Part model, mm, in its own coordinate system. Round coordinates to 2 decimals unless told otherwise and drop trailing zeros. Use CSV: the item, a comma, the result in double quotes. Start each with the question number.
```python
from build123d import *


with BuildPart() as part:
    # Sweep1: sweep along a path in Sketch4
    with BuildLine(Plane.XY) as sweep1_path:
        ThreePointArc((0, 0), (-12.933123295, 3.638699735), (-23.377708341, 12.089525561))
        ThreePointArc((-23.377708341, 12.089525561), (-38.1, 19.05), (-52.822291659, 12.089525561))
        ThreePointArc((-52.822291659, 12.089525561), (-63.266876705, 3.638699735), (-76.2, 0))
    # Sketch2 → Sweep1 (sweep)
    with BuildSketch(Plane(origin=(0, 0, 0), x_dir=(0, 0, -1), z_dir=(1, 0, 0))):
        with BuildLine():
            ThreePointArc((14.885260382, -2.399980647), (0, 2.544792821), (-14.885260382, -2.399980647))
            ThreePointArc((-14.885260382, -2.399980647), (-16.662734914, -2.14232916), (-16.405083427, -0.364854628))
            ThreePointArc((-16.405083427, -0.364854628), (0, 5.084792821), (16.405083427, -0.364854628))
            ThreePointArc((16.405083427, -0.364854628), (16.662734914, -2.14232916), (14.885260382, -2.399980647))
        make_face()
    sweep(path=sweep1_path.line)


solid = part.part
```
1. Drill centre lines: line 1 along X through (y, z) = (7.25, 7); line 2 along Z through (x, y) = (-11.5, 0.5); line 3 along X through (y, z) = (11.75, 13.5). Where is each one in solid material? Low to high. Write a range as [from, to].
2. Band-saw the part on A-A (y = 0.75). Give the number of separate pieces and of enclosed holes in the cut face, then the cut area to 3 significant figures.
3. Flat gauge pins, fed straight in: pin 1 (4 mm diameter, centred on x = -31.5, z = -7.5, fed in from -Y); pin 2 (3 mm diameter, centred on y = 15.5, z = -3, fed in from +X); pin 3 (12 mm diameter, centred on x = -24.5, z = -5, fed in from +Y). Where does each tip first touch, or does it go through?
Answers below:
1,line 1,"x = [-65.35, -60.27], [-15.93, -10.85]"
1,line 2,"z = [-16.58, -14.67], [14.67, 16.58]"
1,line 3,"x = [-55.14, -51.23], [-24.97, -21.06]"
2,separate pieces,"4"
2,enclosed holes,"0"
2,area,"222 mm^2"
3,pin 1,"stops at y = 18.26"
3,pin 2,"stops at x = -18.52"
3,pin 3,"stops at y = 22.61"
